The figure shows three views and two pictorial views of one solid part (mm, origin at its lowest corner). Answer the questions. A direction names the side the tool comes from. Coordinates: 2 decimals unless noted, no trailing zeros. Loops run counter-clockwise (first coordinate to the right, second up) from the corner with the lowest first, then second, coordinate; pieces in that order, holes last. Notation, with made-up numbers: M 38,85 L 58,85 A16 cw 58,112 Z; hole C 42.25,56 d9. An arc over 180 degrees is marked long. One line per item, written item: value. Start each with the question number.
1. Consider probe 1 along X at (y, z) = (12, 30) (1 decimal); probe 2 along X at (y, z) = (5, 30); probe 3 along Z at (x, y) = (30, 14) (1 decimal). Determine where each line is inside the solid, lowest interval first.
2. For the marked faces 4 and 5, determine the directions among +Z, -Z, +X, -X, +Y, -Y from which every point of the face is accessible in a straight line to the end or side of a thin tool.
3. The part is cut by section D-D (y = 22). Write down the section's boundary in (x, z) (1 decimal).
4. Flat-ended cylindrical pins translate along their axes: pin 1 (1.1 mm diameter, centred on y = 5.5, z = 29.5, fed in from +X); pin 2 (1.5 mm diameter, centred on x = 32.5, z = 20, fed in from +Y); pin 3 (1.1 mm diameter, centred on y = 2, z = 30.5, fed in from -X). Find the tip coordinate at first contact, or state that the pin passes through.
5. The part is cut by section B-B (z = 30). State how many separate pieces and enclosed holes the cut face has.
6. The part is cut by section C-C (y = 5). Write down the section's boundary in (x, z).
7. Determine the mould class of the marked faces 1, 2 and 3 for opening direction Z: +Z half, -Z half, draft (parallel to the pull), parting line (faces both ways), or undercut.
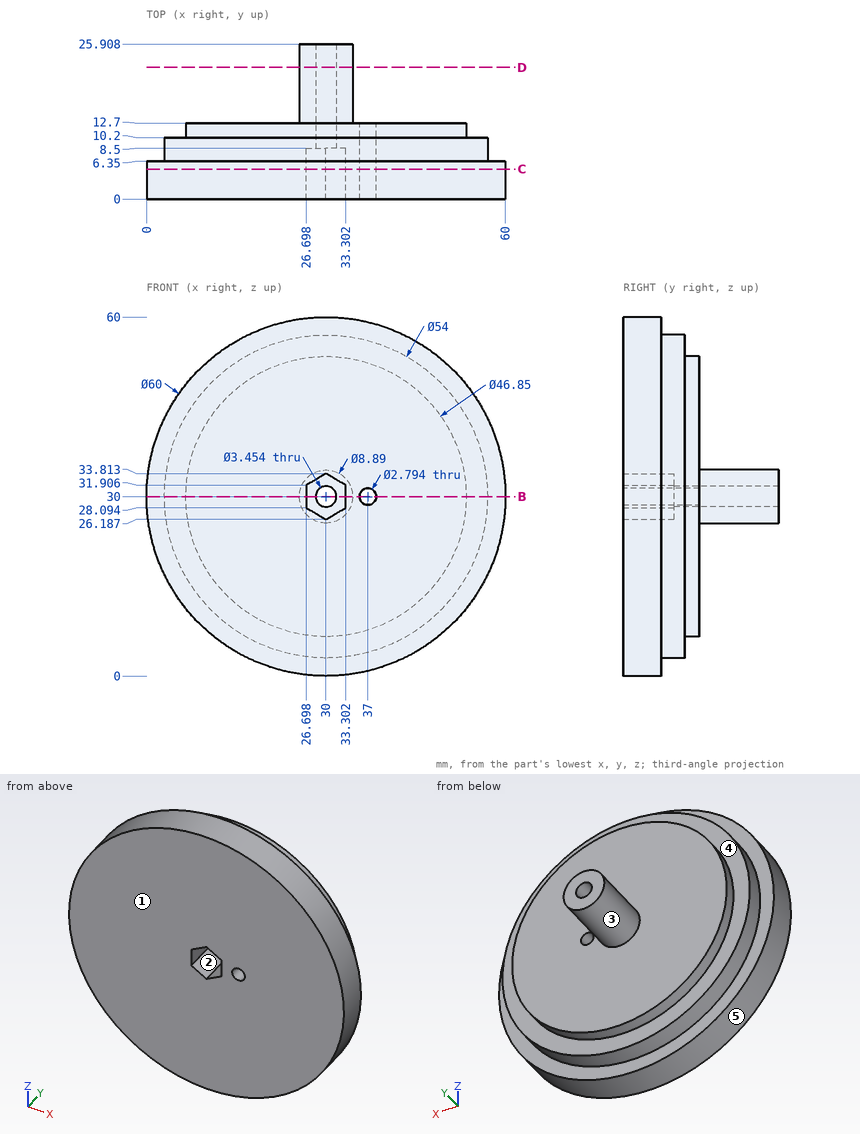
Answer block:
1. probe 1: x = 6.6 to 28.3, 31.7 to 35.6, 38.4 to 53.4
1. probe 2: x = 0 to 26.7, 33.3 to 35.6, 38.4 to 60
1. probe 3: z = 25.6 to 28.3, 31.7 to 34.4
2. face 4: +Y
2. face 5: +Y, -Y
3. outline: C 30,30 d8.9; hole C 30,30 d3.5
4. pin 1: stops at x = 60
4. pin 2: stops at y = 12.7
4. pin 3: stops at x = 0
5. separate pieces: 3
5. enclosed holes: 0
6. outline: C 30,30 d60; hole M 26.7,28.09 L 30,26.19 L 33.3,28.09 L 33.3,31.91 L 30,33.81 L 26.7,31.91 Z; hole C 37,30 d2.79
7. face 1: draft
7. face 2: undercut
7. face 3: parting line
